Part model, mm, in its own coordinate system. Face numbers are marked on the shaded views. A direction names the side the tool comes from. Give positions to 0.01 mm unless a question says otherwise; leave off trailing zeros. Order: outer loops, then holes, each group sorted by start corner. A loop starts at its lowest first (then second) coordinate and runs counter-clockwise, first axis right, second up. Notation, with made-up numbers: M 22,79.5 L 70,79.5 A22 ccw 70,107.5 Z; hole C 88.25,-39.5 d10. An arc over 180 degrees is marked long. One line per question, with ' | ' between items.
```python
from build123d import *

# Parameters (mm, degrees)
SKETCH2_W           = 42.3
SKETCH2_H           = 42.3
BOSS_EXTRUDE1_DEPTH = 39
SKETCH3_R           = 21
BOSS_EXTRUDE2_DEPTH = 48.3
SKETCH4_R           = 4
BOSS_EXTRUDE3_DEPTH = 23.5
SKETCH5_R           = 2.5
BOSS_EXTRUDE4_DEPTH = 9.5
CUT_EXTRUDE1_START  = -2.6
SKETCH6_W           = 3
SKETCH6_H           = 3
CUT_EXTRUDE1_DEPTH  = 14
FILLET1_R           = 1.5
SKETCH7_R           = 2
CUT_EXTRUDE2_DEPTH  = 7


with BuildPart() as part:
    # Sketch2 → Boss-Extrude1 (new body)
    with BuildSketch(Plane(origin=(0, 0, 0), x_dir=(1, 0, 0), z_dir=(0, 1, 0))):
        Rectangle(SKETCH2_W, SKETCH2_H)
    extrude(amount=BOSS_EXTRUDE1_DEPTH)

    # Sketch3 → Boss-Extrude2 (add)
    with BuildSketch(Plane(origin=(0, 39, 0), x_dir=(1, 0, 0), z_dir=(0, 1, 0))):
        with Locations(Location((0, 0, 0), (0, 0, 90))):
            Circle(SKETCH3_R)
    extrude(amount=BOSS_EXTRUDE2_DEPTH)

    # Sketch4 → Boss-Extrude3 (add)
    with BuildSketch(Plane(origin=(0, 87.3, 0), x_dir=(1, 0, 0), z_dir=(0, 1, 0))):
        with Locations(Location((0, 0, 0), (0, 0, 270))):
            Circle(SKETCH4_R)
    extrude(amount=BOSS_EXTRUDE3_DEPTH)

    # Sketch5 → Boss-Extrude4 (add)
    with BuildSketch(Plane.XZ):
        with Locations(Location((0, 0, 0), (0, 0, 270))):
            Circle(SKETCH5_R)
    extrude(amount=BOSS_EXTRUDE4_DEPTH)

    # Sketch6 → Cut-Extrude1 (cut)
    with BuildSketch(Plane(origin=(0, 110.8, 0), x_dir=(1, 0, 0), z_dir=(0, 1, 0)).offset(CUT_EXTRUDE1_START)):
        with Locations((0, 3.7)):
            Rectangle(SKETCH6_W, SKETCH6_H)
    extrude(amount=-CUT_EXTRUDE1_DEPTH, mode=Mode.SUBTRACT)

    # Fillet1
    fillet1_edges = [part.edges().sort_by_distance(p)[0] for p in [
        (1.5, 94.2, -2.954049622),
        (-1.5, 94.2, -2.954049622),
        (1.5, 108.2, -2.954049622),
        (-1.5, 108.2, -2.954049622),
    ]]
    fillet(fillet1_edges, radius=FILLET1_R - 0.0001)  # a hair under: the kernel refuses the full size

    # Sketch7 → Cut-Extrude2 (cut)
    with BuildSketch(Plane(origin=(0, 87.3, 0), x_dir=(1, 0, 0), z_dir=(0, 1, 0))):
        with Locations(Location((0, 17.5, 0), (0, 0, 270))):
            Circle(SKETCH7_R)
        with Locations(Location((17.5, 0, 0), (0, 0, 270))):
            Circle(SKETCH7_R)
        with Locations(Location((0, -17.5, 0), (0, 0, 270))):
            Circle(SKETCH7_R)
        with Locations(Location((-17.5, 0, 0), (0, 0, 270))):
            Circle(SKETCH7_R)
    extrude(amount=-CUT_EXTRUDE2_DEPTH, mode=Mode.SUBTRACT)


solid = part.part
```
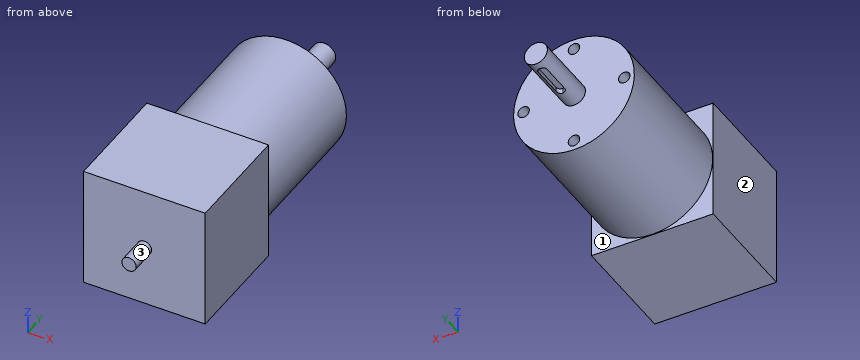
1. Probe L1, parallel to X at y = 86.25, z = 0; L2, parallel to Y at x = 19.5, z = -7.5; L3, parallel to X at y = 82, z = -17.5. List the from-to ranges inside material, lowest first. Write a range as from..to.
Worked out:
L1: x = -21..-19.5, -15.5..15.5, 19.5..21 | L2: y = 0..87.3 | L3: x = -11.61..-2, 2..11.61
2. Slice it at C-C on y = 52. Give the cut face in (x, z).
Worked out:
outline: C 0,0 d42
3. Drop flat-ended pins along their axis: pin 1 (5 mm diameter, centred on x = 17.5, z = 0, fed in from +Y); pin 2 (1.5 mm diameter, centred on y = 70.5, z = 8, fed in from +X); pin 3 (0.8 mm diameter, centred on y = 100.5, z = -3, fed in from +X). Give the stop position or say it passes through.
Worked out:
pin 1: stops at y = 87.3 | pin 2: stops at x = 19.71 | pin 3: stops at x = 3.04
4. Tool access for the marked faces 1, 2 and 3: list every direction of +Z, -Z, +X, -X, +Y, -Y with a clear straight run to the whole face (end or side of a thin tool).
Worked out:
face 1: +Y | face 2: +Z, -Z, -X, +Y, -Y | face 3: -Y
5. Slice it at B-B on x = 17.5. Give the cut face in (y, z).
Worked out:
outline: M 0,-21.15 L 39,-21.15 L 39,-11.61 L 87.3,-11.61 L 87.3,-2 L 80.3,-2 L 80.3,2 L 87.3,2 L 87.3,11.61 L 39,11.61 L 39,21.15 L 0,21.15 Z
6. Slice it at D-D on z = 17.5. Give the cut face in (x, y).
Worked out:
outline: M -21.15,0 L 21.15,0 L 21.15,39 L 11.61,39 L 11.61,87.3 L 2,87.3 L 2,80.3 L -2,80.3 L -2,87.3 L -11.61,87.3 L -11.61,39 L -21.15,39 Z
7. Slice it at A-A on z = 0. Give the cut face in (x, y).
Worked out:
outline: M -21.15,0 L -2.5,0 L -2.5,-9.5 L 2.5,-9.5 L 2.5,0 L 21.15,0 L 21.15,39 L 21,39 L 21,87.3 L 19.5,87.3 L 19.5,80.3 L 15.5,80.3 L 15.5,87.3 L 4,87.3 L 4,110.8 L -4,110.8 L -4,87.3 L -15.5,87.3 L -15.5,80.3 L -19.5,80.3 L -19.5,87.3 L -21,87.3 L -21,39 L -21.15,39 Z
